```python
from build123d import *

# Parameters (mm, degrees)
F0_R     = 7.080456
F1_DEPTH = 1.016
F2_R     = 3.531639
F3_DEPTH = 6.35
F4_R     = 2.582772
F5_DEPTH = 6.35
F6_R     = 7.332478
F7_DEPTH = 1.016


with BuildPart() as f1:
    # F0 (on Top) → F1 (new body)
    with BuildSketch(Plane.XY):
        Circle(F0_R)
    extrude(amount=F1_DEPTH)

    # F2 (on face) → F3 (join)
    with BuildSketch(Plane.XY.offset(1.016)):
        Circle(F2_R)
    extrude(amount=F3_DEPTH)

    # F4 (on face) → F5 (cut)
    with BuildSketch(Plane.XY.offset(7.366)):
        Circle(F4_R)
    extrude(amount=-F5_DEPTH, mode=Mode.SUBTRACT)

    # F6 (on face) → F7 (join)
    with BuildSketch(Plane.XY.offset(7.366)):
        Circle(F6_R)
    extrude(amount=F7_DEPTH)


solid = f1.part
```
Input: part model. Units: mm. Frame: model coordinates. A direction names the side the tool comes from. Give positions to 0.01 mm unless a question says otherwise; leave off trailing zeros. Order: outer loops, then holes, each group sorted by start corner. A loop starts at its lowest first (then second) coordinate and runs counter-clockwise, first axis right, second up.
1. Section C-C on x = -5.75. Return the cut outline in (y, z).
Derived:
outline: (-4.55, 7.37) - (4.55, 7.37) - (4.55, 8.38) - (-4.55, 8.38) - close; (-4.13, 0) - (4.13, 0) - (4.13, 1.02) - (-4.13, 1.02) - close
2. Mould query, pull axis Z, two halves, no side actions, for faces 4 (the cylindrical face through (-5.4, 4.96, 7.87)), 5 (the flat face through (0, 0, 0)), 6 (the flat face through (0, 0, 7.366)). Classes: released by +Z, released by -Z, zero draft, split by the parting line, or undercut.
Derived:
face 4: zero draft
face 5: released by -Z
face 6: undercut
3. Section A-A on x = 0. Return the cut outline in (y, z), and give its area (3 significant figures).
Derived:
outline: (-7.33, 7.37) - (-3.53, 7.37) - (-3.53, 1.02) - (-7.08, 1.02) - (-7.08, 0) - (7.08, 0) - (7.08, 1.02) - (3.53, 1.02) - (3.53, 7.37) - (7.33, 7.37) - (7.33, 8.38) - (-7.33, 8.38) - close; hole (-2.58, 1.02) - (2.58, 1.02) - (2.58, 7.37) - (-2.58, 7.37) - close
area: 41.3 mm2
4. Reachability of faces 1 (the flat face through (0, 0, 1.016)), 2 (the flat face through (0, 0, 8.382)), 3 (the cylindrical face through (6.753, 2.127, 0.501)) from +Z, -Z, +X, -X, +Y, -Y: full face, straight path, thin tool, end or side. Return the list, or none.
Derived:
face 1: none
face 2: +Z, +X, -X, +Y, -Y
face 3: -Z
5. Pin query (flat end, axial travel): pin 1 (4 mm diameter, centred on x = 2.5, z = 2, fed in from +Y); pin 2 (3 mm diameter, centred on x = -5, z = 1.5, fed in from -Y); pin 3 (3 mm diameter, centred on y = 3, z = 7, fed in from -X). Return the tip coordinate at first contact, or that it passes through.
Derived:
pin 1: stops at y = 7.04
pin 2: stops at y = -6.11
pin 3: stops at x = -7.17
6. Material intervals for L1, parallel to Z at x = 2.25, y = -1; L2, parallel to Y at x = 0, z = 5.5; L3, parallel to Y at x = -0.5, z = 6.75, sorted ascending.
Derived:
L1: z = 0 to 1.02, 7.37 to 8.38
L2: y = -3.53 to -2.58, 2.58 to 3.53
L3: y = -3.5 to -2.53, 2.53 to 3.5
7. Section B-B on y = 4. Return the cut outline in (x, z).
Derived:
outline: (-6.15, 7.37) - (6.15, 7.37) - (6.15, 8.38) - (-6.15, 8.38) - close; (-5.84, 0) - (5.84, 0) - (5.84, 1.02) - (-5.84, 1.02) - close
